from build123d import *

# Parameters (mm, degrees)
SKETCH1_R           = 4.765
BOSS_EXTRUDE1_DEPTH = 9.5
SKETCH3_W           = 9.43
SKETCH3_H           = 9.43
CUT_EXTRUDE1_DEPTH  = 36.900947063
CUT_EXTRUDE2_DEPTH  = 36.900947063
SKETCH5_R           = 1.59
CUT_EXTRUDE3_DEPTH  = 36.682899346
CHAMFER1_SIZE       = 2.54
CHAMFER1_SIZE_2     = 7.62
CHAMFER2_SIZE       = 7.62
CHAMFER2_SIZE_2     = 2.54


with BuildPart() as part:
    # Sketch1 → Boss-Extrude1 (new, symmetric)
    with BuildSketch(Plane.XY):
        with BuildLine():
            Line((0, 9.77), (-22.23, 9.77))
            Line((-22.23, 9.77), (-22.23, 4.77))
            Line((-22.23, 4.77), (-9.711509246, -1.067468107))
            ThreePointArc((-9.711509246, -1.067468107), (-5.877874817, -7.804068659), (1.655323868, -9.628748771))
            Line((1.655323868, -9.628748771), (28.58, -5))
            Line((28.58, -5), (28.58, 0))
            Line((28.58, 0), (9.77, 0))
            ThreePointArc((9.77, 0), (6.908433252, 6.908433252), (0, 9.77))
        make_face()
        Circle(SKETCH1_R, mode=Mode.SUBTRACT)
    extrude(amount=BOSS_EXTRUDE1_DEPTH, both=True)

    # Sketch3 → Cut-Extrude1 (cut, through all)
    with BuildSketch(Plane(origin=(0, 9.77, 0), x_dir=(1, 0, 0), z_dir=(0, 1, 0))):
        with Locations((-17.515, 0)):
            Rectangle(SKETCH3_W, SKETCH3_H)
        with Locations((23.865, 0)):
            Rectangle(SKETCH3_W, SKETCH3_H)
    extrude(amount=-CUT_EXTRUDE1_DEPTH, mode=Mode.SUBTRACT)

    # Sketch4 → Cut-Extrude2 (cut, through all)
    with BuildSketch(Plane(origin=(0, 9.77, 0), x_dir=(1, 0, 0), z_dir=(0, 1, 0))):
        with BuildLine():
            Line((-3.91, 5.08), (6.25, 5.08))
            ThreePointArc((6.25, 5.08), (11.33, 0), (6.25, -5.08))
            Line((6.25, -5.08), (-3.91, -5.08))
            ThreePointArc((-3.91, -5.08), (-8.99, 0), (-3.91, 5.08))
        make_face()
    extrude(amount=-CUT_EXTRUDE2_DEPTH, mode=Mode.SUBTRACT)

    # Sketch5 → Cut-Extrude3 (cut, through all)
    with BuildSketch(Plane.XY.offset(9.5)):
        with Locations((-19.69, 7.23)):
            Circle(SKETCH5_R)
        with Locations((26.04, -2.54)):
            Circle(SKETCH5_R)
    extrude(amount=-CUT_EXTRUDE3_DEPTH, mode=Mode.SUBTRACT)

    # Chamfer1
    # the kernel refuses this chamfer: 7.62, 2.54 mm, written as the material it takes off along each edge
    with BuildSketch(Plane(origin=(-22.23, 29.544364901, -9.5), x_dir=(-0.1090261201798072, 0, 0.9940388851139267), z_dir=(0, -1, 0))) as chamfer1_piece_1:
        Polygon((CHAMFER1_SIZE * 0.994038885114, -CHAMFER1_SIZE * 0.10902612018), (-CHAMFER1_SIZE_2 * 0.10902612018, -CHAMFER1_SIZE_2 * 0.994038885114), (0, 0), align=None)
    extrude(amount=44.548729802, mode=Mode.SUBTRACT)
    with BuildSketch(Plane(origin=(28.58, -24.774364901, -9.5), x_dir=(-0.9999257509361695, 0, -0.012185754582199181), z_dir=(0, 1, 0))) as chamfer1_piece_2:
        Polygon((CHAMFER1_SIZE_2 * 0.999925750936, CHAMFER1_SIZE_2 * 0.0121857545822), (-CHAMFER1_SIZE * 0.0121857545822, CHAMFER1_SIZE * 0.999925750936), (0, 0), align=None)
    extrude(amount=44.548729802, mode=Mode.SUBTRACT)

    # Chamfer2
    # the kernel refuses this chamfer: 7.62, 2.54 mm, written as the material it takes off along each edge
    with BuildSketch(Plane(origin=(-22.23, 29.544364901, 9.5), x_dir=(0.9999257509361695, 0, 0.012185754582199181), z_dir=(0, -1, 0)), Plane(origin=(28.58, -24.774364901, 9.5), x_dir=(-0.9999257509361695, 0, 0.012185754582199181), z_dir=(0, 1, 0))) as chamfer2_piece_1:
        Polygon((CHAMFER2_SIZE * 0.999925750936, -CHAMFER2_SIZE * 0.0121857545822), (-CHAMFER2_SIZE_2 * 0.0121857545822, -CHAMFER2_SIZE_2 * 0.999925750936), (0, 0), align=None)
    extrude(amount=44.548729802, mode=Mode.SUBTRACT)


solid = part.part
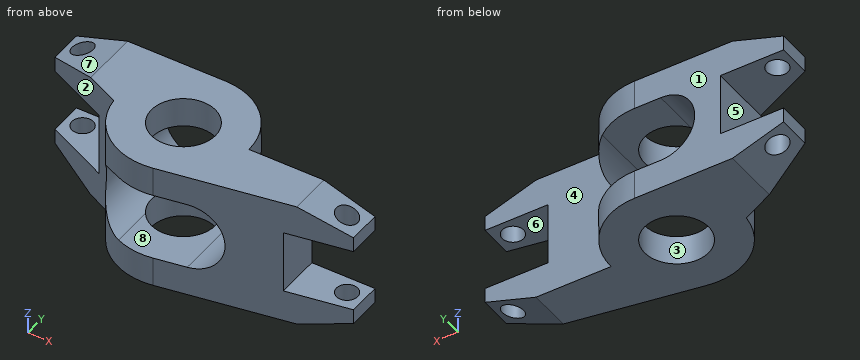
The model under review builds one solid part; all positions refer to its coordinate system, in mm. Face numbers are marked on the shaded views. A direction names the side the tool comes from. Round coordinates to 2 decimals unless told otherwise and drop trailing zeros. Loops run counter-clockwise (first coordinate to the right, second up) from the corner with the lowest first, then second, coordinate; pieces in that order, holes last. Notation, with made-up numbers: M -6.75,-31 L -1.75,-31 A19 ccw -1.75,-6 Z; hole C 81,55 d5. An arc over 180 degrees is marked long. Answer as a JSON object with one key per item and string values.
Item 1: For line 1 along Z through (x, y) = (8, -4.5); line 2 along X through (y, z) = (7.23, -6.85); line 3 along X through (y, z) = (-1.25, 0.25), list the stretches that pass through material, from the lowest coordinate up.
Check sheet entries:
{"line 1": "-9.5 to -4.77, 4.77 to 9.5", "line 2": "-22.23 to -21.28, -18.1 to 6.57", "line 3": "-9.69 to -8.98, 11.32 to 19.15"}
Item 2: We need section A-A, the plane y = -2. State how many separate pieces and enclosed holes the cut face has, and give its area (3 significant figures).
Check sheet entries:
{"separate pieces": "4", "enclosed holes": "0", "area": "337 mm2"}
Item 3: We need section D-D, the plane x = 3.5. State the section outline as (y, z) points.
Check sheet entries:
{"outline": "M -9.31,-9.5 L -3.23,-9.5 L -3.23,-5.08 L -9.31,-5.08 Z; M -9.31,5.08 L -3.23,5.08 L -3.23,9.5 L -9.31,9.5 Z; M 3.23,-9.5 L 9.12,-9.5 L 9.12,-5.08 L 3.23,-5.08 Z; M 3.23,5.08 L 9.12,5.08 L 9.12,9.5 L 3.23,9.5 Z"}
Item 4: We need section B-B, the plane z = 0. State the section outline as (x, y) points, and give its area (3 significant figures).
Check sheet entries:
{"outline": "M -12.8,0.37 L -9.71,-1.07 A9.77 ccw -8.99,-3.83 L -8.99,9.77 L -12.8,9.77 Z; M 11.33,-7.97 L 19.15,-6.62 L 19.15,0 L 11.33,0 Z", "area": "97.3 mm2"}
Item 5: The part is to be moulded in two halves that separate along X. For the marked faces 1, 2 and 3, say which applies: +X half, -X half, draft (parallel to the pull), parting line (faces both ways), or undercut.
Check sheet entries:
{"face 1": "draft", "face 2": "-X half", "face 3": "undercut"}
Item 6: Tool access review of the marked faces 4, 5, 6, 7 and 8: name each direction out of +Z, -Z, +X, -X, +Y, -Y from which nothing blocks a thin tool from reaching the whole face with its end or side.
Check sheet entries:
{"face 4": "+Z, -Z, +X, +Y", "face 5": "-X, +Y, -Y", "face 6": "+X, +Y, -Y", "face 7": "+Z, -X, +Y, -Y", "face 8": "+Y, -Y"}
Item 7: We need section C-C, the plane y = 8. State the section outline as (x, z) points (3 decimals).
Check sheet entries:
{"outline": "M -22.23,-6.96 L -21.081,-7.343 L -21.081,-4.715 L -22.23,-4.715 Z; M -22.23,4.715 L -21.081,4.715 L -21.081,7.343 L -22.23,6.96 Z; M -18.299,-8.27 L -14.61,-9.5 L 5.608,-9.5 L 5.608,-5.08 L -3.91,-5.08 A5.08 cw -3.91,5.08 L 5.608,5.08 L 5.608,9.5 L -14.61,9.5 L -18.299,8.27 L -18.299,4.715 L -12.8,4.715 L -12.8,-4.715 L -18.299,-4.715 Z"}
Item 8: Clearance check with flat-ended pins moving along their axes: P1, Ø2, axis at y = 4, z = 6, coming from the -X side; P2, Ø7.5, axis at x = -19, y = 6.5, coming from the +Z side; P3, Ø6, axis at y = 0.5, z = -7.5, coming from the -X side; P4, Ø5, axis at x = -19.69, y = 7.23, coming from the -Z side. State where each tip first meets the part, or that it passes through.
Check sheet entries:
{"P1": "x = -22.23", "P2": "z = 9.29", "P3": "x = -19.51", "P4": "z = -8.64"}
